from build123d import *

# Parameters (mm, degrees)
SKETCH_1_W               = 25
SKETCH_1_H               = 25
SKETCH_1_W_2             = 19
SKETCH_1_H_2             = 19
EXTRUDE_1_DEPTH          = 280
SKETCH_2_R               = 3
SKETCH_2_R_2             = 2
CUT_EXTRUDE_1_DEPTH      = 283.223315833
CUT_EXTRUDE_2_DEPTH      = 283.223315833
CUT_EXTRUDE_2_DEPTH_BACK = 283.223315833
SKETCH_3_R               = 1.5


with BuildPart() as part:
    # 草图1 → 凸台-拉伸1 (new body)
    with BuildSketch(Plane(origin=(0, 0, 0), x_dir=(1, 0, 0), z_dir=(0, 1, 0))):
        with Locations((12.5, 12.5)):
            Rectangle(SKETCH_1_W, SKETCH_1_H)
        with Locations((12.5, 12.5)):
            Rectangle(SKETCH_1_W_2, SKETCH_1_H_2, mode=Mode.SUBTRACT)
    extrude(amount=EXTRUDE_1_DEPTH)

    # 草图2 → 切除-拉伸1 (cut, through all)
    with BuildSketch(Plane(origin=(0, 0, 0), x_dir=(0, 0, -1), z_dir=(1, 0, 0))):
        with Locations(Location((12.5, 10, 0), (0, 0, 180))):
            Circle(SKETCH_2_R)
        with Locations(Location((12.5, 40, 0), (0, 0, 180))):
            Circle(SKETCH_2_R)
        with Locations(Location((12.5, 70, 0), (0, 0, 180))):
            Circle(SKETCH_2_R)
        with Locations(Location((17, 140, 0), (0, 0, 180))):
            Circle(SKETCH_2_R_2)
        with Locations(Location((8, 140, 0), (0, 0, 180))):
            Circle(SKETCH_2_R_2)
    extrude(amount=CUT_EXTRUDE_1_DEPTH, mode=Mode.SUBTRACT)

    # 草图3 → 切除-拉伸2 (cut, two sides: drawn at the far end of the back side and taken through both)
    with BuildSketch(Plane.XY.offset(-CUT_EXTRUDE_2_DEPTH_BACK)):
        with Locations((6, 180)):
            Circle(SKETCH_3_R)
        with Locations((6, 215)):
            Circle(SKETCH_3_R)
    extrude(amount=CUT_EXTRUDE_2_DEPTH + CUT_EXTRUDE_2_DEPTH_BACK, mode=Mode.SUBTRACT)


solid = part.part
CAD build for the part. Positions are in the model's coordinates, mm. A direction names the side the tool comes from. Give positions to 0.01 mm unless a question says otherwise; leave off trailing zeros. Order: outer loops, then holes, each group sorted by start corner. A loop starts at its lowest first (then second) coordinate and runs counter-clockwise, first axis right, second up. Notation, with made-up numbers: (64.5, 63.25) - (87.5, 63.25) arc R32 ccw to (87.5, 95.25) - close; hole circle Ø1 at (55.25, 75). An arc over 180 degrees is marked (long way). Write each question's results on one line, items separated by ' | '.
1. 3-axis set-ups, long thin cutter, end or side, ignore diameter. For faces 5 (the face through (23.48, 37.97, -14.71)), 6 (the face through (12, 138, -3)): which of +Z, -Z, +X, -X, +Y, -Y reach the whole face in a straight line?
Calculated:
face 5: +X, -X | face 6: +Y, -Y
2. Probe L1, parallel to Y at x = 1.55, z = -12.5; L2, parallel to Y at x = 6, z = -23.9; L3, parallel to X at y = 84.5, z = -6. List the from-to ranges inside material, lowest first. Write a range as from..to.
Calculated:
L1: y = 0..7, 13..37, 43..67, 73..280 | L2: y = 0..178.5, 181.5..213.5, 216.5..280 | L3: x = 0..3, 22..25
3. Saw through at B-B on y = 191.5. List the corners of the cut face in (x, z).
Calculated:
outline: (0, -25) - (25, -25) - (25, 0) - (0, 0) - close; hole (3, -22) - (22, -22) - (22, -3) - (3, -3) - close
4. Pull direction Y, two halves, no side cores. Call faces 1 (the face through (3, 138, -12)), 2 (the face through (1.48, 37.97, -14.71)), 3 (the face through (23, 280, -13)), 4 (the face through (1.48, 7.97, -14.71)): released by +Y, released by -Y, zero draft, split by the parting line, or undercut.
Calculated:
face 1: zero draft | face 2: undercut | face 3: released by +Y | face 4: undercut
5. Saw through at A-A on x = 18.5. List the corners of the cut face in (y, z), and give its area (3 significant figures).
Calculated:
outline: (0, -25) - (280, -25) - (280, -22) - (0, -22) - close; (0, -3) - (280, -3) - (280, 0) - (0, 0) - close | area: 1,680 mm2
